Geometry: final body of the model. Coordinates: model frame, mm. Face numbers are marked on the shaded views. A direction names the side the tool comes from. Round coordinates to 2 decimals unless told otherwise and drop trailing zeros. Loops run counter-clockwise (first coordinate to the right, second up) from the corner with the lowest first, then second, coordinate; pieces in that order, holes last. Notation, with made-up numbers: (-8, -31.75) -> (17, -31.75) arc R26 cw to (17, -8.75) -> close; hole circle Ø6 at (82.5, 32.25). An arc over 180 degrees is marked (long way). Answer in a Markdown table with one row per item.
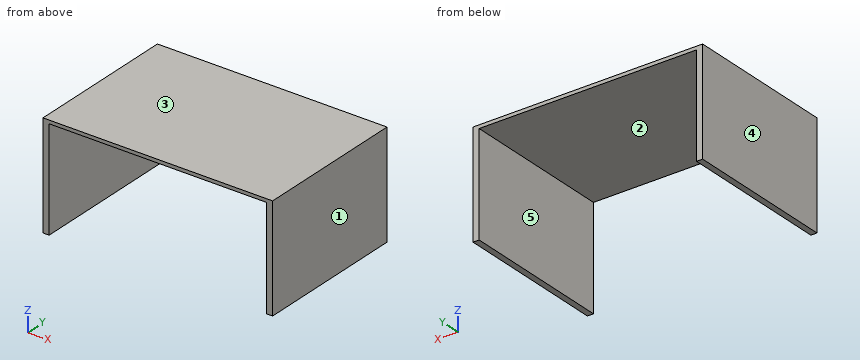
```python
from build123d import *

# Parameters (mm, degrees)
BOSS_EXTRUDE1_DEPTH = 45


with BuildPart() as part:
    # Sketch1 → Boss-Extrude1 (new body)
    with BuildSketch(Plane.XZ.offset(-155)):
        Polygon((-195.2, 13), (-197, 13), (-197, 43), (-261, 43), (-261, 13), (-262.8, 13), (-262.8, 44), (-195.2, 44), align=None)
    extrude(amount=BOSS_EXTRUDE1_DEPTH)


solid = part.part
```
Item 1: Mould query, pull axis X, two halves, no side actions, for the marked faces 1, 2 and 3. Classes: released by +X, released by -X, zero draft, split by the parting line, or undercut.
Ans:
| item | result |
|---|---|
| face 1 | released by +X |
| face 2 | undercut |
| face 3 | zero draft |
Item 2: Section query A-A, the plane z = 22. Output: boundary loops of the cut face in (x, y), and give its area (3 significant figures).
Ans:
| item | result |
|---|---|
| outline | (-262.8, 110) -> (-261, 110) -> (-261, 155) -> (-262.8, 155) -> close; (-197, 110) -> (-195.2, 110) -> (-195.2, 155) -> (-197, 155) -> close |
| area | 162 mm2 |
Item 3: Ray query, L1, parallel to X at y = 148, z = 15.5; L2, parallel to Z at x = -203.5, y = 113. Return the intervals inside material, ascending.
Ans:
| item | result |
|---|---|
| L1 | -262.8 to -261, -197 to -195.2 |
| L2 | 43 to 44 |
Item 4: Set-up query: the marked faces 4 and 5. Return all of +Z, -Z, +X, -X, +Y, -Y with unobstructed straight access to the full face (end or side cutting, diameter ignored); none if empty.
Ans:
| item | result |
|---|---|
| face 4 | +Z, -Z, -X, +Y, -Y |
| face 5 | -Z, +Y, -Y |
Item 5: Section query B-B, the plane y = 145. Output: boundary loops of the cut face in (x, z).
Ans:
| item | result |
|---|---|
| outline | (-262.8, 13) -> (-261, 13) -> (-261, 43) -> (-197, 43) -> (-197, 13) -> (-195.2, 13) -> (-195.2, 44) -> (-262.8, 44) -> close |
Item 6: First-contact query: P1, Ø2, axis at x = -235.5, y = 132, coming from the -Z side. Flat tip, straight axial feed; report the tip coordinate or a pass-through.
Ans:
| item | result |
|---|---|
| P1 | z = 43 |
Item 7: Section query C-C, the plane x = -198.5. Output: boundary loops of the cut face in (y, z), and give its area (3 significant figures).
Ans:
| item | result |
|---|---|
| outline | (110, 43) -> (155, 43) -> (155, 44) -> (110, 44) -> close |
| area | 45.0 mm2 |
